The figure shows three views and two pictorial views of one solid part (mm, origin at its lowest corner). Answer the questions. A direction names the side the tool comes from. Coordinates: 2 decimals unless noted, no trailing zeros. Loops run counter-clockwise (first coordinate to the right, second up) from the corner with the lowest first, then second, coordinate; pieces in that order, holes last. Notation, with made-up numbers: M 50.5,16.25 L 66.5,16.25 A31 cw 66.5,45.25 Z; hole C 33,65 d5. An arc over 180 degrees is marked long. Answer in a Markdown table with one row per item. Add a question column.
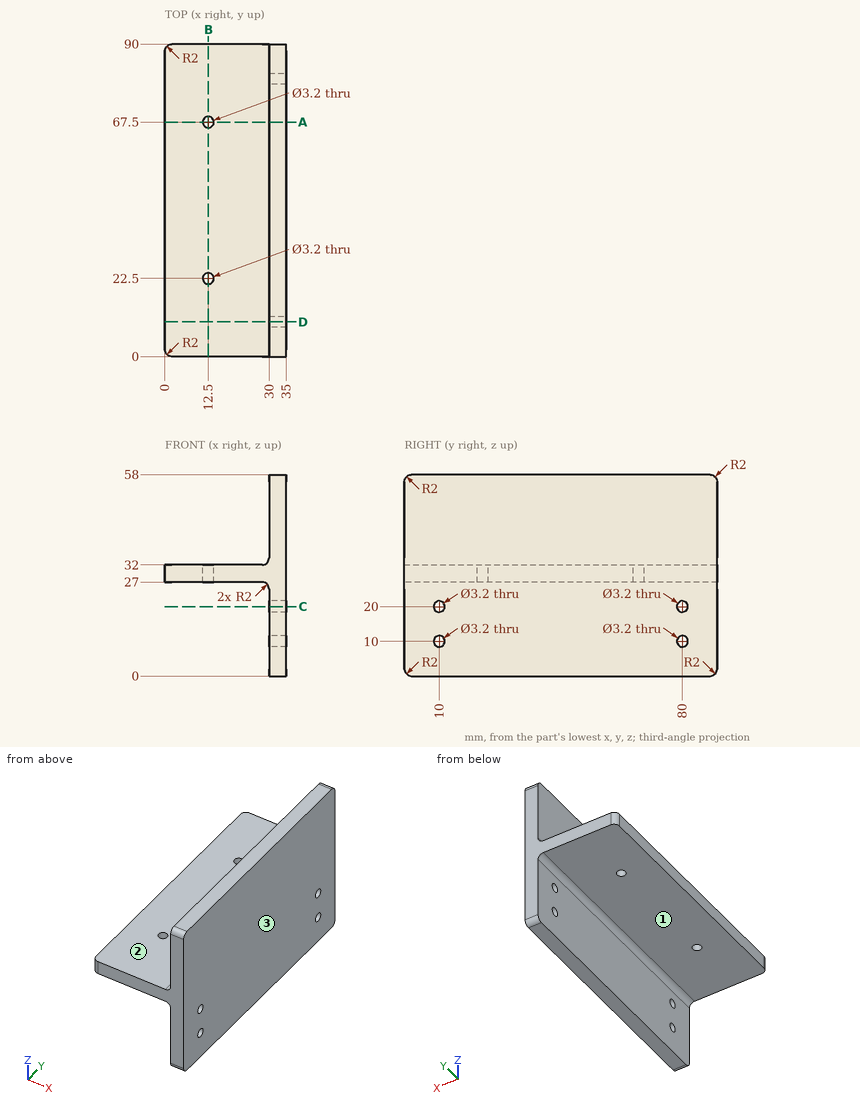
(1) A cutting plane is placed at C-C (z = 20). Give the vertices of the cut face in (x, y), plus the area to 3 significant figures.
(2) A cutting plane is placed at D-D (y = 10). Give the vertices of the cut face in (x, z), plus the area to 3 significant figures.
(3) Straight lines are drawn through the part: line 1 (Z direction, x = 33, y = 80); line 2 (Y direction, x = 12, z = 28); line 3 (X direction, y = 67.5, z = 30.45). For each, find the intervals that lie inside material, in ascending order.
(4) A cutting plane is placed at A-A (y = 67.5). Give the vertices of the cut face in (x, z), plus the area to 3 significant figures.
(5) For the marked faces 1, 2 and 3, determine the directions among +Z, -Z, +X, -X, +Y, -Y from which every point of the face is accessible in a straight line to the end or side of a thin tool.
(6) Each of these flat-tipped pins is pushed along its axis until it touches: pin 1 (3 mm diameter, centred on x = 11, y = 58.5, fed in from +Z); pin 2 (10 mm diameter, centred on x = 13.5, y = 17, fed in from -Z); pin 3 (3.5 mm diameter, centred on y = 10, z = 10, fed in from -X). Where does it stop, or does it pass through?
(7) A cutting plane is placed at B-B (x = 12.5). Give the vertices of the cut face in (y, z).
Solved:
| question | item | result |
|---|---|---|
| 1 | outline | M 30,0 L 35,0 L 35,8.4 L 30,8.4 Z; M 30,11.6 L 35,11.6 L 35,78.4 L 30,78.4 Z; M 30,81.6 L 35,81.6 L 35,90 L 30,90 Z |
| 1 | area | 418 mm² |
| 2 | outline | M 0,27 L 28,27 A2 cw 30,25 L 30,21.6 L 35,21.6 L 35,58 L 30,58 L 30,34 A2 cw 28,32 L 0,32 Z; M 30,0 L 35,0 L 35,8.4 L 30,8.4 Z; M 30,11.6 L 35,11.6 L 35,18.4 L 30,18.4 Z |
| 2 | area | 410 mm² |
| 3 | line 1 | z = 0 to 8.4, 11.6 to 18.4, 21.6 to 58 |
| 3 | line 2 | y = 0 to 20.98, 24.02 to 65.98, 69.02 to 90 |
| 3 | line 3 | x = 0 to 10.9, 14.1 to 35 |
| 4 | outline | M 0,27 L 10.9,27 L 10.9,32 L 0,32 Z; M 14.1,27 L 28,27 A2 cw 30,25 L 30,0 L 35,0 L 35,58 L 30,58 L 30,34 A2 cw 28,32 L 14.1,32 Z |
| 4 | area | 426 mm² |
| 5 | face 1 | -Z, -X, +Y, -Y |
| 5 | face 2 | +Z, -X, +Y, -Y |
| 5 | face 3 | +Z, -Z, +X, +Y, -Y |
| 6 | pin 1 | stops at z = 32 |
| 6 | pin 2 | stops at z = 27 |
| 6 | pin 3 | stops at x = 30 |
| 7 | outline | M 0,27 L 20.9,27 L 20.9,32 L 0,32 Z; M 24.1,27 L 65.9,27 L 65.9,32 L 24.1,32 Z; M 69.1,27 L 90,27 L 90,32 L 69.1,32 Z |
